Solid Edge part; units mm, degrees
sketch "Sketch1" plane through (0, 0, 0) normal (0, 0, 1) x (1, 0, 0)
  line L0 (0, 0) -> (42.5, 0)
  line L1 (42.5, 0) -> (42.5, 80)
  line L2 (42.5, 80) -> (0, 80)
  line L3 (0, 80) -> (0, 0)
extrude "Protrusion1" add sketch "Sketch1" along normal blind 1
sketch "Sketch2" plane through (21.25, 40, 1) normal (0, 0, 1) x (1, 0, 0)
  line L0 (-20, 40) -> (-20, -40)
  line L1 (-20, -40) -> (20, -40)
  line L2 (20, -40) -> (20, 40)
  line L3 (20, 40) -> (-20, 40)
extrude "Vysunutí_2" add sketch "Sketch2" along normal blind 1
sketch "Sketch3" plane through (21.25, 40, 2) normal (0, 0, 1) x (1, 0, 0)
  line L0 (-22.5, -40) -> (22.5, -40)
  line L1 (22.5, -40) -> (22.5, 40)
  line L2 (22.5, 40) -> (-22.5, 40)
  line L3 (-22.5, 40) -> (-22.5, -40)
extrude "Vysunutí_3" add sketch "Sketch3" along normal blind 1
sketch "Sketch4" plane through (21.25, 40, 3) normal (0, 0, 1) x (1, 0, 0)
  line L0 (-22.5, 75) -> (-22.5, 40)
  line L1 (-22.5, 40) -> (22.5, 40)
  line L2 (22.5, 40) -> (-12.5, 75)
  line L3 (-22.5, 75) -> (-12.5, 75)
extrude "Protrusion2" add sketch "Sketch4" against normal blind 16
sketch "Sketch5" plane through (21.25, 57.5, 3) normal (0, 0, 1) x (0, -1, 0)
  line L0 (-23.75, 21.25) -> (-23.75, -22.5)
  line L1 (-23.75, -22.5) -> (-57.5, -22.5)
  line L2 (-57.5, -22.5) -> (-57.5, -12.5)
  line L3 (-57.5, -12.5) -> (-23.75, 21.25)
extrude "Cutout1" cut sketch "Sketch5" against normal blind 15
sketch "Sketch6" plane through (21.25, 97.5, -13) normal (0, 0, -1) x (0, -1, 0)
  line L0 (-15, 12.5) -> (-7.6278, 5.1278)
  line L1 (-7.6278, 5.1278) -> (16.25, -18.75)
  line L2 (17.5, -20) -> (16.25, -18.75)
  line L3 (17.5, 22.5) -> (17.5, -20)
  line L4 (16.25, 22.5) -> (17.5, 22.5)
  line L5 (16.25, 22.5) -> (-15, 22.5)
  line L6 (-17.5, 22.5) -> (-15, 22.5)
  line L7 (-17.5, 15) -> (-17.5, 22.5)
  line L8 (-15, 12.5) -> (-17.5, 15)
extrude "Vysunutí_6" add sketch "Sketch6" along normal blind 1
sketch "Sketch7" plane through (20, 96.25, -14) normal (0, 0, -1) x (-1, 0, 0)
  line L0 (21.25, 16.25) -> (21.25, 17.5)
  line L1 (21.25, 18.75) -> (21.25, 17.5)
  line L2 (12.25, 18.75) -> (21.25, 18.75)
  line L3 (11, 17.5) -> (12.25, 18.75)
  line L4 (9.75, 16.25) -> (11, 17.5)
  line L5 (9.75, 16.25) -> (-22.75, -16.25)
  line L6 (-22.75, -16.25) -> (-21.25, -16.25)
  line L7 (21.25, -16.25) -> (-21.25, -16.25)
  line L8 (21.25, 16.25) -> (21.25, -16.25)
extrude "Vysunutí_7" add sketch "Sketch7" along normal blind 1
sketch "Sketch8" plane through (21.25, 40.625, 3) normal (0, 0, 1) x (1, 0, 0)
  line L0 (22.5, -40.625) -> (-22.5, -40.625)
  line L1 (-22.5, -40.625) -> (-22.5, -37.625)
  line L2 (-22.5, -37.625) -> (22.5, -37.625)
  line L3 (22.5, -37.625) -> (22.5, -40.625)
extrude "Cutout2" cut sketch "Sketch8" against normal blind 3
The listing builds one solid part. Answer for the finished solid, in the listing's coordinates (mm). A direction names the side the tool comes from. Coordinates: 2 decimals unless noted, no trailing zeros. Loops run counter-clockwise (first coordinate to the right, second up) from the corner with the lowest first, then second, coordinate; pieces in that order, holes last. Notation, with made-up numbers: M 60,-20.5 L 77,-20.5 A10 cw 77,-4.5 Z; hole C -7.5,24.5 d3. An arc over 180 degrees is marked long. Answer in a Markdown table with one row per item.
1) Find section A-A (x = 11). Determine the outline of the cut face in (y, z).
Answers below:
| item | result |
|---|---|
| outline | M 3,0 L 80,0 L 80,-15 L 111.75,-15 L 111.75,-14 L 110.25,-14 L 110.25,-13 L 112.75,-13 L 112.75,-12 L 81.25,-12 L 81.25,3 L 3,3 Z |
2) Find section B-B (y = 99). Determine the outline of the cut face in (x, z).
Answers below:
| item | result |
|---|---|
| outline | M -1.25,-15 L 23.75,-15 L 23.75,-14 L 22.25,-14 L 22.25,-13 L 24.75,-13 L 24.75,-12 L -1.25,-12 Z |
3) Which of the six approach directions +Z, -Z, +X, -X, +Y, -Y give full straight-line access (tool end or side, diameter ignored) to faces 4 (the flat face through (21, 81.25, -4)), 5 (the flat face through (25, 98, -13)), 6 (the flat face through (25.495, 97.255, -14.493))?
Answers below:
| item | result |
|---|---|
| face 4 | +Z, +X, -X, +Y |
| face 5 | +X, +Y |
| face 6 | -Z, +X, +Y |
4) Find section C-C (x = 16.5). Determine the outline of the cut face in (y, z).
Answers below:
| item | result |
|---|---|
| outline | M 3,0 L 80,0 L 80,-15 L 106.25,-15 L 106.25,-14 L 104.75,-14 L 104.75,-13 L 107.25,-13 L 107.25,-12 L 81.25,-12 L 81.25,3 L 3,3 Z |
5) Given pin 1 (2 mm diameter, centred on x = 0.5, y = 51.5, fed in from -Z); pin 2 (1.1 mm diameter, centred on y = 44.5, z = 0.5, fed in from -X); pin 3 (1.5 mm diameter, centred on x = 24, z = -2.5, fed in from +Y), each flat-ended and moving along its own axis, determine where each tip first touches the part or whether it passes through.
Answers below:
| item | result |
|---|---|
| pin 1 | z = 0 |
| pin 2 | x = 0 |
| pin 3 | y = 81.25 |
6) Find the intervals of material crossed by probe 1 along Z at (x, y) = (26, 51.5); probe 2 along Z at (x, y) = (3.5, 82); probe 3 along Y at (x, z) = (23.5, -3), in increasing order.
Answers below:
| item | result |
|---|---|
| probe 1 | 0 to 3 |
| probe 2 | -15 to -12 |
| probe 3 | 80 to 81.25 |
7) Determine the mould class of faces 1 (the flat face through (0, 42, 2)), 2 (the flat face through (21, 42, 0)), 3 (the flat face through (31.52, 92.23, -12.67)) for opening direction Z: released by +Z, released by -Z, zero draft, split by the parting line, or undercut.
Answers below:
| item | result |
|---|---|
| face 1 | undercut |
| face 2 | released by -Z |
| face 3 | zero draft |
8) Find section D-D (z = -8.5). Determine the outline of the cut face in (x, y).
Answers below:
| item | result |
|---|---|
| outline | M -1.25,80 L 43.75,80 L 42.5,81.25 L -1.25,81.25 Z |
